Design review of the part built by this model. Coordinates are the model's own, in mm. Face numbers are marked on the shaded views. A direction names the side the tool comes from. Give positions to 0.01 mm unless a question says otherwise; leave off trailing zeros. Write each loop counter-clockwise with the first axis right and the second up, starting at its lowest first coordinate (ties: lowest second). Pieces come first, ordered by that corner, then holes. Notation, with made-up numbers: (22.5, 80) -> (58.5, 80) arc R20 cw to (58.5, 99) -> close; hole circle Ø11 at (-4.5, 84.5). An arc over 180 degrees is marked (long way). Use CSV: the item, a comma, the result in double quotes.
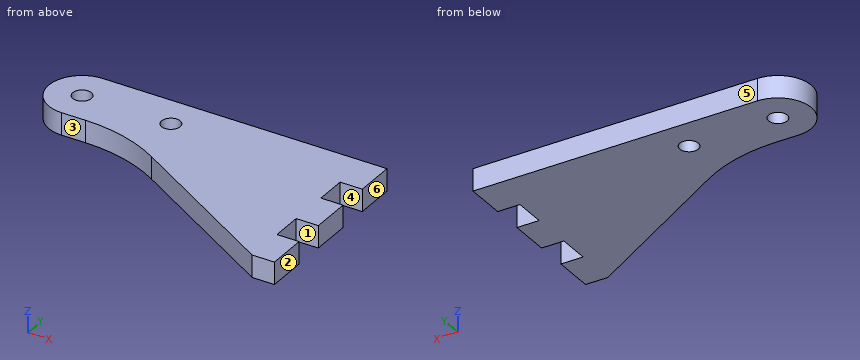
Autodesk Inventor part; units mm, degrees
ref_plane "YZ Plane" through (0, 0, 0) normal (1, 0, 0) x (0, 1, 0)
ref_plane "XZ Plane" through (0, 0, 0) normal (0, 1, 0) x (-1, 0, 0)
ref_plane "XY Plane" through (0, 0, 0) normal (0, 0, 1) x (1, 0, 0)
sketch "Sketch1" plane through (0, 0, 0) normal (0, 0, 1) x (1, 0, 0)
  line L0 (-20, -7.5) -> (-5, -7.5)
  line L1 (44, 7.5) -> (-20, 7.5)
  arc A0 (-20, 7.5) -> (-20, -7.5) centre (-20, 0) ccw
  circle A1 centre (-20, 0) radius 2.1
  line L2 (44, 7.5) -> (44, -1.5)
  line L3 (39, -1.5) -> (39, -8.5)
  line L4 (39, -8.5) -> (44, -8.5)
  line L5 (44, -8.5) -> (44, -17.5)
  line L6 (44, -17.5) -> (39, -17.5)
  line L7 (39, -1.5) -> (44, -1.5)
  circle A2 centre (0, 0) radius 2.1
  line L8 (39, -17.5) -> (39, -24.5)
  line L9 (39, -24.5) -> (44, -24.5)
  line L10 (44, -24.5) -> (44, -33.5)
  line L11 (44, -33.5) -> (39, -33.5)
  line L12 (39, -33.5) -> (-5, -7.5)
  dimension "d1" = 4.2
  dimension "d8" = 15
  dimension "d9" = 5
  dimension "d10" = 7
  dimension "d11" = 9
  dimension "d12" = 9
  dimension "d14" = 4.2
  dimension "d15" = 20
  dimension "d16" = 64
  dimension "d17" = 15
  dimension "d18" = 7
  dimension "d19" = 9
extrude "Extrusion1" add sketch "Sketch1" along normal blind 5
fillet "Fillet1" radius 35 1 edges at (-5, -7.5, 2.5)
equation "\"d1\" = d14"
equation "\"d12\" = d11"
equation "\"d18\" = d10"
equation "\"d19\" = d12"
properties part number "gate-upper-link"
(1) Take a section at D-D (x = 0). Write out the cut boundary in (y, z).
Established:
outline,"(-10.68, 0) -> (-2.1, 0) -> (-2.1, 5) -> (-10.68, 5) -> close; (2.1, 0) -> (7.5, 0) -> (7.5, 5) -> (2.1, 5) -> close"
(2) Mouldability with a two-part tool opening along Y and no side actions: class the marked faces 4, 5 and 6 as +Y half, -Y half, draft (parallel to the pull), parting line (faces both ways), or undercut.
Established:
face 4,"undercut"
face 5,"+Y half"
face 6,"draft"
(3) Take a section at B-B (y = 0). Write out the cut boundary in (x, z).
Established:
outline,"(-27.5, 0) -> (-22.1, 0) -> (-22.1, 5) -> (-27.5, 5) -> close; (-17.9, 0) -> (-2.1, 0) -> (-2.1, 5) -> (-17.9, 5) -> close; (2.1, 0) -> (44, 0) -> (44, 5) -> (2.1, 5) -> close"
(4) Clearance check with a flat-ended pin moving along its axis: pin 1 (2.5 mm diameter, centred on y = -6, z = 2, fed in from +X). State where the tip first meets the part, or that it passes through.
Established:
pin 1,"stops at x = 39"
(5) Tool access review of the marked faces 1, 2 and 3: name each direction out of +Z, -Z, +X, -X, +Y, -Y from which nothing blocks a thin tool from reaching the whole face with its end or side.
Established:
face 1,"+Z, -Z, +X"
face 2,"+Z, -Z, +X, +Y, -Y"
face 3,"+Z, -Z, -X, -Y"
(6) Take a section at A-A (x = 40.5). Write out the cut boundary in (y, z).
Established:
outline,"(-33.5, 0) -> (-24.5, 0) -> (-24.5, 5) -> (-33.5, 5) -> close; (-17.5, 0) -> (-8.5, 0) -> (-8.5, 5) -> (-17.5, 5) -> close; (-1.5, 0) -> (7.5, 0) -> (7.5, 5) -> (-1.5, 5) -> close"
(7) Take a section at C-C (z = 2.1). Write out the cut boundary in (x, y).
Established:
outline,"(-20, -7.5) -> (-14.57, -7.5) arc R35 cw to (3.24, -12.37) -> (39, -33.5) -> (44, -33.5) -> (44, -24.5) -> (39, -24.5) -> (39, -17.5) -> (44, -17.5) -> (44, -8.5) -> (39, -8.5) -> (39, -1.5) -> (44, -1.5) -> (44, 7.5) -> (-20, 7.5) arc R7.5 ccw to start; hole circle Ø4.2 at (-20, 0); hole circle Ø4.2 at (0, 0)"
(8) For line 1 along X through (y, z) = (-6, 0.5); line 2 along Y through (x, z) = (0, 2.5); line 3 along Y through (x, z) = (13, 3.95), list the stretches that pass through material, from the lowest coordinate up. Write a range as [from, to].
Established:
line 1,"x = [-24.5, 39]"
line 2,"y = [-10.68, -2.1], [2.1, 7.5]"
line 3,"y = [-18.14, 7.5]"
